Check sheet for the modelled part. Datum: model origin and axes. Units: mm. A direction names the side the tool comes from. Round coordinates to 2 decimals unless told otherwise and drop trailing zeros. Loops run counter-clockwise (first coordinate to the right, second up) from the corner with the lowest first, then second, coordinate; pieces in that order, holes last. Notation, with made-up numbers: (8.25, 6.5) - (32.25, 6.5) arc R19 ccw to (32.25, 24.5) - close; hole circle Ø2 at (-8.5, 46). An arc over 180 degrees is marked (long way). Put each result on its own line as item: value. Start each with the question number.
Item 1: Section check C-C, the plane x = 51. Record the cut outline in (y, z).
Item 2: Material ranges on line 1 along Z through (x, y) = (-17, 2); line 2 along X through (y, z) = (13, 14); line 3 along Z through (x, y) = (-39, 16.5), recorded low to high.
Item 3: Section check B-B, the plane z = -51. Record the cut outline in (x, y), and give its area (3 significant figures).
Item 4: Section check A-A, the plane y = -4.5. Record the cut outline in (x, z), and give its area (3 significant figures).
Item 5: Tool access check on faces 1 (the flat face through (-5, -2, 67.353)), 2 (the flat face through (-5, 22.86, -1)), 3 (the flat face through (-71.16, 0, -3)). Record the directions out of +Z, -Z, +X, -X, +Y, -Y that give a thin tool (end or side, any length) a straight path to the whole face; none if there is none.
Item 6: Section check D-D, the plane z = -35. Record the cut outline in (x, y), and give its area (3 significant figures).
Item 7: Draft check along Y on faces 4 (the flat face through (-12, 15.335, -59)), 5 (the flat face through (-5, 25.4, -1)), 6 (the flat face through (45.873, -1, -59)). Enter one of: pulls with the +Y half, pulls with the -Y half, needs draft (parallel to the pull), parting line crosses it, or undercut.
Item 8: Gauge pin test, flat ends, axial feed: pin 1 Ø5 at (x, z) = (-18, -42.5) entering from -Y; pin 2 Ø11.5 at (x, z) = (-3, -61) entering from -Y; pin 3 Ø20.5 at (x, z) = (-9, -53) entering from -Y. Record the tip position at first contact, or that the pin passes through.
from build123d import *

# Parameters (mm, degrees)
F0_W          = 133.6063072085
F0_H          = 144.1496908665
F1_DEPTH      = 25.4
F1_DEPTH_BACK = 25.4
F2_T          = -2.54
F3_W          = 114.4931351459
F3_H          = 32.4011910707
F4_DEPTH      = 25.4
F5_T          = -2.54


# Not quite as in the source:
# - a shell that OpenCascade refuses in one call is made with other operations: the cavity is built on its own and cut out


with BuildPart() as f1:
    # F0 (on Front) → F1 (new body, two sides)
    with BuildSketch(Plane.XZ) as f1_sk:
        with Locations((-4.3567232788, -2.181828022)):
            Rectangle(F0_W, F0_H)
    extrude(amount=F1_DEPTH)
    extrude(f1_sk.sketch, amount=-F1_DEPTH_BACK)

    # F2
    f2_openings = [f1.faces().sort_by_distance(p)[0] for p in [
        (-4.356723, -25.4, -2.181828),
    ]]
    offset(amount=F2_T, openings=f2_openings)

    # F3 (on face) → F4 (join)
    with BuildSketch(Plane.XY.offset(-71.7166734552)):
        with Locations((-11.3733093101, -0.8654547855)):
            Rectangle(F3_W, F3_H)
    extrude(amount=F4_DEPTH)

    # F5: a shell. OpenCascade refuses it in one call, so the cavity is built on its own and cut out:
    # the body offset inwards by the wall thickness, plus a prism from it out through each open face.
    f5_core = offset(f1.part, amount=F5_T, kind=Kind.INTERSECTION, mode=Mode.PRIVATE)
    f5_exits = [f5_core.faces().sort_by_distance(p)[0] for p in [
        (-12.643309, -14.52605, -60.286673),
    ]]
    add(f5_core, mode=Mode.SUBTRACT)
    extrude(f5_exits, amount=-F5_T, mode=Mode.SUBTRACT)


solid = f1.part
Check result:
1. outline: (-25.4, -74.26) - (25.4, -74.26) - (25.4, 69.89) - (-25.4, 69.89) - (-25.4, 67.35) - (22.86, 67.35) - (22.86, -71.72) - (-25.4, -71.72) - close
2. line 1: -74.26 to -71.72, -48.86 to -46.32, 67.35 to 69.89
2. line 2: -71.16 to -68.62, 59.91 to 62.45
2. line 3: -74.26 to -71.72, 67.35 to 69.89
3. outline: (-71.16, -25.4) - (-68.62, -25.4) - (-68.62, 12.8) - (43.33, 12.8) - (43.33, -17.07) - (45.87, -17.07) - (45.87, 15.34) - (-68.62, 15.34) - (-68.62, 22.86) - (59.91, 22.86) - (59.91, -25.4) - (62.45, -25.4) - (62.45, 25.4) - (-71.16, 25.4) - close
3. area: 951 mm²
4. outline: (-71.16, -74.26) - (62.45, -74.26) - (62.45, 69.89) - (-71.16, 69.89) - close; hole (-68.62, -71.72) - (43.33, -71.72) - (43.33, -48.86) - (-68.62, -48.86) - close; hole (-68.62, -46.32) - (45.87, -46.32) - (45.87, -71.72) - (59.91, -71.72) - (59.91, 67.35) - (-68.62, 67.35) - close
4. area: 1,730 mm²
5. face 1: -Y
5. face 2: none
5. face 3: +Z, -Z, -X, +Y, -Y
6. outline: (-71.16, -25.4) - (-68.62, -25.4) - (-68.62, 22.86) - (59.91, 22.86) - (59.91, -25.4) - (62.45, -25.4) - (62.45, 25.4) - (-71.16, 25.4) - close
6. area: 585 mm²
7. face 4: undercut
7. face 5: pulls with the +Y half
7. face 6: needs draft
8. pin 1: y = 22.86
8. pin 2: y = 12.8
8. pin 3: y = -17.07
